```python
from build123d import *

# Parameters (mm, degrees)
SKETCH1_R           = 11.1
BOSS_EXTRUDE1_DEPTH = 58
SKETCH2_R           = 24.777888598
SKETCH2_R_2         = 10
CUT_EXTRUDE1_DEPTH  = 24
CUT_EXTRUDE2_START  = -44
SKETCH2_2_R         = 24.777888598
SKETCH2_2_R_2       = 10
CUT_EXTRUDE2_DEPTH  = 14
SKETCH4_R           = 10
BOSS_EXTRUDE3_DEPTH = 30
SKETCH5_R           = 10
BOSS_EXTRUDE4_DEPTH = 45
SKETCH6_R           = 10
CUT_EXTRUDE3_DEPTH  = 12
SKETCH7_R           = 8.287445099
CUT_EXTRUDE4_DEPTH  = 122


with BuildPart() as part:
    # Sketch1 → Boss-Extrude1 (new body)
    with BuildSketch(Plane.XY):
        Circle(SKETCH1_R)
    extrude(amount=BOSS_EXTRUDE1_DEPTH)

    # Sketch2 → Cut-Extrude1 (cut)
    with BuildSketch(Plane(origin=(0, 0, 0), x_dir=(-1, 0, 0), z_dir=(0, 0, -1))):
        Circle(SKETCH2_R)
        Circle(SKETCH2_R_2, mode=Mode.SUBTRACT)
    extrude(amount=-CUT_EXTRUDE1_DEPTH, mode=Mode.SUBTRACT)

    # Sketch2_2 → Cut-Extrude2 (cut)
    with BuildSketch(Plane(origin=(0, 0, 0), x_dir=(-1, 0, 0), z_dir=(0, 0, -1)).offset(CUT_EXTRUDE2_START)):
        Circle(SKETCH2_2_R)
        Circle(SKETCH2_2_R_2, mode=Mode.SUBTRACT)
    extrude(amount=-CUT_EXTRUDE2_DEPTH, mode=Mode.SUBTRACT)

    # Sketch4 → Boss-Extrude3 (add)
    with BuildSketch(Plane.XY.offset(58)):
        Circle(SKETCH4_R)
    extrude(amount=BOSS_EXTRUDE3_DEPTH)

    # Sketch5 → Boss-Extrude4 (add)
    with BuildSketch(Plane(origin=(0, 0, 0), x_dir=(-1, 0, 0), z_dir=(0, 0, -1))):
        Circle(SKETCH5_R)
    extrude(amount=BOSS_EXTRUDE4_DEPTH)

    # Sketch6 → Cut-Extrude3 (cut)
    with BuildSketch(Plane(origin=(0, 0, -45), x_dir=(-1, 0, 0), z_dir=(0, 0, -1))):
        Circle(SKETCH6_R)
    extrude(amount=-CUT_EXTRUDE3_DEPTH, mode=Mode.SUBTRACT)

    # Sketch7 → Cut-Extrude4 (cut, through all)
    with BuildSketch(Plane(origin=(0, 0, -33), x_dir=(-1, 0, 0), z_dir=(0, 0, -1))):
        Circle(SKETCH7_R)
    extrude(amount=-CUT_EXTRUDE4_DEPTH, mode=Mode.SUBTRACT)


solid = part.part
```
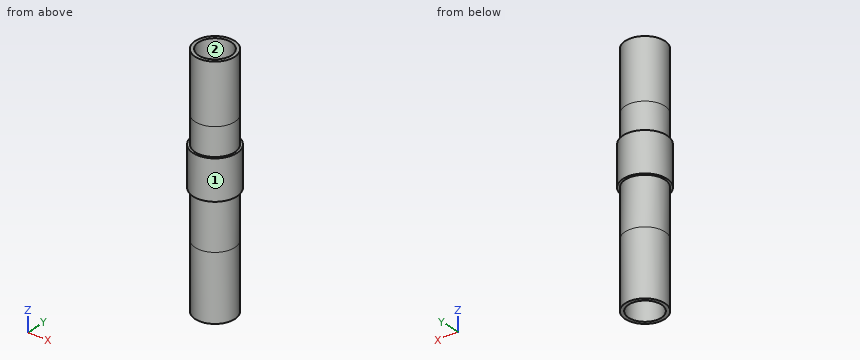
Build history of the part. All positions in model axes, mm. Face numbers are marked on the shaded views. Round coordinates to 2 decimals unless told otherwise and drop trailing zeros. Loops run counter-clockwise (first coordinate to the right, second up) from the corner with the lowest first, then second, coordinate; pieces in that order, holes last.
Item 1: Saw through at C-C (z = 80). List the corners of the cut face in (x, y).
Item 2: Drill centre lines: line 1 along Y through (x, z) = (0, 47); line 2 along Z through (x, y) = (-9.5, -3.5); line 3 along X through (y, z) = (-6.75, 30). Where is each one in solid material? Low to high.
Item 3: Pin check, flat tip, straight feed: P1, Ø6, axis at x = -6.5, z = -19, coming from the -Y side. Stop position of the tip, or through.
Item 4: Saw through at A-A (x = 0). List the corners of the cut face in (y, z).
Item 5: Two-plate mould, pull along Y, no slides. Class the marked faces 1 and 2: released by +Y, released by -Y, zero draft, split by the parting line, or undercut.
Worked answers:
1. outline: circle Ø20 at (0, 0); hole circle Ø16.57 at (0, 0)
2. line 1: y = -10 to -8.29, 8.29 to 10
2. line 2: z = 24 to 44
2. line 3: x = -8.81 to -4.81, 4.81 to 8.81
3. P1: stops at y = -9.37
4. outline: (-11.1, 24) - (-10, 24) - (-10, -33) - (-8.29, -33) - (-8.29, 88) - (-10, 88) - (-10, 44) - (-11.1, 44) - close; (8.29, -33) - (10, -33) - (10, 24) - (11.1, 24) - (11.1, 44) - (10, 44) - (10, 88) - (8.29, 88) - close
5. face 1: split by the parting line
5. face 2: undercut
